from build123d import *

# Parameters (mm, degrees)
ESQUISSE1_R                  = 2.4999999999999893
ESQUISSE1_R_2                = 1.1499999999999992
EXTRUSION1_DEPTH             = 5
ESQUISSE1_R_3                = 2.5000000000000027
EXTRUSION1_2_DEPTH           = 5
EXTRUSION2_DEPTH             = 18
EXTRUSION3_DEPTH             = 2.5
ENL_V_MAT_EXTRU_1_DEPTH      = 39.32538157223775
ENL_V_MAT_EXTRU_1_DEPTH_BACK = 39.32538157223775
ESQUISSE4_R                  = 2.749999999999997
ESQUISSE4_R_2                = 2.749999999999998
CONG_3_R                     = 2
ENL_V_MAT_EXTRU_3_DEPTH      = 102.20266619760267
ENL_V_MAT_EXTRU_5_DEPTH      = 106.71602432156358
ENL_V_MAT_EXTRU_6_REACH      = 81.21
CONG_4_R                     = 6
CONG_5_R                     = 6
ESQUISSE9_R                  = 1.100000000000001
ESQUISSE9_R_2                = 1.0999999999999992
ENL_V_MAT_EXTRU_7_DEPTH      = 6


with BuildPart() as part:
    # Esquisse1 → Extrusion1 (new body)
    with BuildSketch(Plane.XY):
        with Locations((20.851873368125936, -74.73281291154764)):
            Circle(ESQUISSE1_R)
        with Locations((20.851873368125936, -74.73281291154764)):
            Circle(ESQUISSE1_R_2, mode=Mode.SUBTRACT)
    extrude(amount=EXTRUSION1_DEPTH)



with BuildPart() as body_2:
    # Esquisse1 → Extrusion1 2 (new body)
    with BuildSketch(Plane.XY):
        with Locations((-21.148126631874074, -74.73281291154764)):
            Circle(ESQUISSE1_R_3)
        with Locations((-21.148126631874074, -74.73281291154764)):
            Circle(ESQUISSE1_R_2, mode=Mode.SUBTRACT)
    extrude(amount=EXTRUSION1_2_DEPTH)


with BuildPart() as body_3:
    # Esquisse2 → Extrusion2 (new, symmetric)
    with BuildSketch(Plane(origin=(0, 0, 0), x_dir=(0, 0, -1), z_dir=(1, 0, 0))):
        Polygon((-16.664409805958893, -94.72524914650984), (-16.664409805958893, -78.97076866014885), (-7.5846798827186035, -78.97076866014885), (0, -72.23281291154765), (17.904062513857752, -57.96690094689117), (21.643440589343484, -57.97016684873832), (21.641519151826778, -60.17016600966495), (13.695222620932038, -67.54623887711948), align=None)
    extrude(amount=EXTRUSION2_DEPTH, both=True)


with BuildPart() as part_1:
    add(part.part)

    add(body_2.part)  # Extrusion3 merges body 2

    add(body_3.part)  # Extrusion3 merges body 3
    # Esquisse3 → Extrusion3 (add)
    with BuildSketch(Plane.XY.offset(2.5)):
        with BuildLine():
            Line((-23.15262617413516, -73.23883112281155), (-22.298126631874073, -73.23883112281155))
            Line((-22.298126631874073, -73.23883112281155), (-22.298126631874073, -74.73281291154764))
            ThreePointArc((-22.298126631874073, -74.73281291154764), (-21.148126631874074, -75.88281291154763), (-19.998126631874076, -74.73281291154764))
            Line((-19.998126631874076, -74.73281291154764), (-19.998126631874076, -73.23883112281155))
            Line((-19.998126631874076, -73.23883112281155), (-19.143627089612984, -73.23883112281155))
            Line((-19.143627089612984, -73.23883112281155), (-16.812156322257874, -73.23883112281158))
            Line((-16.812156322257874, -73.23883112281158), (-16.8121563222579, -77.23281291154763))
            Line((-16.8121563222579, -77.23281291154763), (-21.148126631874074, -77.23281291154764))
            ThreePointArc((-21.148126631874074, -77.23281291154764), (-23.382511834993743, -75.85420613610354), (-23.15262617413516, -73.23883112281155))
        make_face()
        with BuildLine():
            Line((18.847373825864864, -73.23883112281155), (19.701873368125938, -73.23883112281155))
            Line((19.701873368125938, -73.23883112281155), (19.701873368125938, -74.73281291154764))
            ThreePointArc((19.701873368125938, -74.73281291154764), (20.851873368125936, -75.88281291154763), (22.001873368125935, -74.73281291154764))
            Line((22.001873368125935, -74.73281291154764), (22.001873368125935, -73.23883112281155))
            Line((22.001873368125935, -73.23883112281155), (22.85637291038701, -73.23883112281155))
            ThreePointArc((22.85637291038701, -73.23883112281155), (23.0862585712456, -75.85420613610351), (20.85187336812597, -77.23281291154763))
            Line((20.85187336812597, -77.23281291154763), (16.59665054376802, -77.23281291154761))
            Line((16.59665054376802, -77.23281291154761), (16.59665054376802, -73.23883112281155))
            Line((16.59665054376802, -73.23883112281155), (18.847373825864864, -73.23883112281155))
        make_face()
    extrude(amount=EXTRUSION3_DEPTH)

    # Esquisse4 → Enlèv. mat.-Extru.1 (cut, two sides: drawn at the far end of the back side and taken through both)
    with BuildSketch(Plane(origin=(0, -78.97076866014885, 0), x_dir=(-1, 0, 0), z_dir=(0, 1, 0)).offset(-ENL_V_MAT_EXTRU_1_DEPTH_BACK)):
        with Locations(Location((-9.992794939980836, 11.38535169586409, 0), (0, 0, 270))):
            Circle(ESQUISSE4_R)
        with Locations(Location((0.00720473933372518, 11.382819165765587, 0), (0, 0, 270))):
            Circle(ESQUISSE4_R_2)
        with Locations(Location((10.007204418648286, 11.380286635667082, 0), (0, 0, 270))):
            Circle(ESQUISSE4_R_2)
    extrude(amount=ENL_V_MAT_EXTRU_1_DEPTH + ENL_V_MAT_EXTRU_1_DEPTH_BACK, mode=Mode.SUBTRACT)

    # Congé3
    cong_3_edges = [part_1.edges().sort_by_distance(p)[0] for p in [
        (-16.812156322257874, -73.23883112281158, 3.75),
        (16.59665054376802, -73.23883112281155, 3.75),
    ]]
    fillet(cong_3_edges, radius=CONG_3_R)

    # Esquisse6 → Enlèv. mat.-Extru.3 (cut, through all)
    with BuildSketch(Plane.XY.offset(5)):
        with BuildLine():
            Line((19.701873368125938, -73.23883112281155), (18.847373825864864, -73.23883112281155))
            ThreePointArc((18.847373825864864, -73.23883112281155), (20.851873368125936, -72.23281291154765), (22.85637291038701, -73.23883112281155))
            Line((22.85637291038701, -73.23883112281155), (22.001873368125935, -73.23883112281155))
            Line((22.001873368125935, -73.23883112281155), (22.001873368125935, -74.73281291154764))
            ThreePointArc((22.001873368125935, -74.73281291154764), (20.851873368125936, -75.88281291154763), (19.701873368125938, -74.73281291154764))
            Line((19.701873368125938, -74.73281291154764), (19.701873368125938, -73.23883112281155))
        make_face()
        with BuildLine():
            Line((-19.143627089612988, -73.23883112281155), (-19.998126631874076, -73.23883112281155))
            Line((-19.998126631874076, -73.23883112281155), (-19.998126631874076, -74.73281291154764))
            ThreePointArc((-19.998126631874076, -74.73281291154764), (-21.148126631874074, -75.88281291154763), (-22.298126631874073, -74.73281291154764))
            Line((-22.298126631874073, -74.73281291154764), (-22.298126631874073, -73.23883112281155))
            Line((-22.298126631874073, -73.23883112281155), (-23.15262617413516, -73.23883112281155))
            ThreePointArc((-23.15262617413516, -73.23883112281155), (-21.148126631874074, -72.23281291154764), (-19.143627089612988, -73.23883112281155))
        make_face()
    extrude(amount=-ENL_V_MAT_EXTRU_3_DEPTH, mode=Mode.SUBTRACT)

    # Esquisse7 → Enlèv. mat.-Extru.5 (cut, through all)
    with BuildSketch(Plane(origin=(18, 0, 0), x_dir=(0, 0, -1), z_dir=(1, 0, 0))):
        Polygon((22.38759689084557, -59.06637403320253), (18.619915990338253, -59.06637403320253), (2.127272735037141, -72.00940646483387), (2.127272735037142, -79.68956966642843), (22.38759689084557, -60.215467045024496), align=None)
    extrude(amount=-ENL_V_MAT_EXTRU_5_DEPTH, mode=Mode.SUBTRACT)

    # Enlèv. mat.-Extru.6: up to this plane
    enl_v_mat_extru_6_end = Plane(origin=(-23.648126631874074, -59.06637403320253, -18.619915990338253), z_dir=(0, 0.7866767496715903, 0.6173651201081433))
    # Esquisse8 → Enlèv. mat.-Extru.6 (cut, up to the surface)
    with BuildSketch(Plane(origin=(0, -44.301458010279546, -39.66022266935793), x_dir=(1, 0, 0), z_dir=(0, -0.745056791328178, -0.6670010327546427)), mode=Mode.PRIVATE) as enl_v_mat_extru_6_sk1:
        Polygon((16.22439568808015, 59.743411480582274), (-16.434037279491676, 59.74341148058227), (-16.43403727949168, 40.55997816141156), (16.22439568808015, 40.559978161411564), align=None)
    enl_v_mat_extru_6_tool1 = split(extrude(enl_v_mat_extru_6_sk1.sketch, amount=-ENL_V_MAT_EXTRU_6_REACH, mode=Mode.PRIVATE), bisect_by=enl_v_mat_extru_6_end, keep=Keep.BOTH, mode=Mode.PRIVATE)
    add(enl_v_mat_extru_6_tool1.solids().sort_by_distance((-0.104821, -77.75269, -2.294362))[0], mode=Mode.SUBTRACT)

    # Congé4
    cong_4_edges = [part_1.edges().sort_by_distance(p)[0] for p in [
        (-17.217018639745838, -77.90227429690431, -2.127272735037141),
        (17.112197844040075, -77.90227429690431, -2.127272735037141),
    ]]
    fillet(cong_4_edges, radius=CONG_4_R)

    # Congé5
    cong_5_edges = [part_1.edges().sort_by_distance(p)[0] for p in [
        (-18, -86.84800890332934, 16.664409805958893),
        (18, -86.84800890332934, 16.664409805958893),
    ]]
    fillet(cong_5_edges, radius=CONG_5_R)

    # Esquisse9 → Enlèv. mat.-Extru.7 (cut)
    with BuildSketch(Plane(origin=(0, -78.97076866014885, 0), x_dir=(-1, 0, 0), z_dir=(0, 1, 0))):
        with Locations(Location((-16, 9.584679882718603, 0), (0, 0, 90))):
            Circle(ESQUISSE9_R)
        with Locations(Location((16, 9.584679882718603, 0), (0, 0, 90))):
            Circle(ESQUISSE9_R_2)
    extrude(amount=-ENL_V_MAT_EXTRU_7_DEPTH, mode=Mode.SUBTRACT)


solid = part_1.part
Build history of the part. All positions in model axes, mm. A direction names the side the tool comes from. Give positions to 0.01 mm unless a question says otherwise; leave off trailing zeros. Order: outer loops, then holes, each group sorted by start corner. A loop starts at its lowest first (then second) coordinate and runs counter-clockwise, first axis right, second up. Notation, with made-up numbers: M 20,39.5 L 35,39.5 A31 cw 35,78.5 Z; hole C 2,84 d6. An arc over 180 degrees is marked long. Use one line per item in the form item = value.
Q1. Wall check: probe 1 along X at (y, z) = (-80, 11); probe 2 along Y at (x, z) = (5.5, 5.5); probe 3 along Z at (x, y) = (-10, -80). Give the ranges that are in metal, low to high.
Conclusion:
probe_1 = -17.99 to -12.73, -7.28 to -2.73, 2.72 to 7.27, 12.72 to 17.99
probe_2 = -84.73 to -83.43, -78 to -77.12
probe_3 = 8.05 to 8.63, 14.13 to 16.66
Q2. Pin check, flat tips, straight feed: P1, Ø10, axis at x = -0.5, y = -71.5, coming from the +Z side; P2, Ø8, axis at x = -6.5, z = 6.5, coming from the -Y side; P3, Ø2.5, axis at x = -16, z = 9.58, coming from the +Y side; P4, Ø12, axis at y = -73.5, z = -4.5, coming from the -X side. Stop position of each tip, or through.
Conclusion:
P1 = 4.8
P2 = -89.21
P3 = -78.97
P4 = -23.65
Q3. Pull direction Z, two halves, no side cores. Call faces 1 (the flat face through (-17, -74, -2.127)), 2 (the flat face through (0, -87, 16.664)), 3 (the cylindrical face through (-0.13, -84.35, 14.13)): released by +Z, released by -Z, zero draft, split by the parting line, or undercut.
Conclusion:
face_1 = released by -Z
face_2 = released by +Z
face_3 = undercut
Q4. Slice it at A-A, the plane x = -8. Write the cut outline in (y, z).
Conclusion:
outline = M -94.73,16.66 L -91.68,13.26 L -78.97,13.26 L -78.97,16.66 Z; M -88.31,9.5 L -84.15,4.85 L -80.24,8.36 L -59.07,-18.62 L -59.07,-21.64 L -57.97,-21.64 L -57.97,-17.9 L -72.23,0 L -78.97,7.58 L -78.97,9.5 Z
Q5. Which spindle directions (+Z, -Z, +X, -X, +Y, -Y) get a long thin tool onto all of the face, cutting with end or side? Do faces 4 (the flat face through (0, -59.066, -20)), 5 (the flat face through (19, -77.233, 4)), 6 (the flat face through (0, -78.971, 15)), 7 (the flat face through (20.8, -76.1, 0)), 8 (the flat face through (-16.434, -79, 3)). Say none if no direction does.
Conclusion:
face_4 = -Z, +X, -X, -Y
face_5 = +Z, -Z, +X, -Y
face_6 = +Z, +X, -X, +Y
face_7 = -Z, +X, +Y, -Y
face_8 = -Z
Q6. Slice it at B-B, the plane z = 12. Write the cut outline in (x, y).
Conclusion:
outline = M -17.85,-90.55 L -12.69,-90.55 L -12.69,-78.97 L -17.85,-78.97 Z; M -7.33,-90.55 L -2.69,-90.55 L -2.69,-78.97 L -7.33,-78.97 Z; M 2.67,-90.55 L 7.31,-90.55 L 7.31,-78.97 L 2.67,-78.97 Z; M 12.67,-90.55 L 17.85,-90.55 L 17.85,-78.97 L 12.67,-78.97 Z
Q7. Slice it at D-D, the plane x = 8. Write the cut outline in (y, z), and give its area (3 significant figures).
Conclusion:
outline = M -94.73,16.66 L -91.7,13.28 L -78.97,13.28 L -78.97,16.66 Z; M -88.3,9.49 L -84.15,4.85 L -80.24,8.36 L -59.07,-18.62 L -59.07,-21.64 L -57.97,-21.64 L -57.97,-17.9 L -72.23,0 L -78.97,7.58 L -78.97,9.49 Z
area = 111 mm2
Q8. Slice it at C-C, the plane y = -83. Write the cut outline in (x, z), and give its area (3 significant figures).
Conclusion:
outline = M -18,3.57 L -16.43,3.57 L -16.43,5.88 L 16.22,5.88 L 16.22,3.57 L 18,3.57 L 18,10.66 A6 ccw 12,16.66 L -12,16.66 A6 ccw -18,10.66 Z; hole C -16,9.58 d2.2; hole C -10.01,11.38 d5.5; hole C -0.01,11.38 d5.5; hole C 9.99,11.39 d5.5; hole C 16,9.58 d2.2
area = 302 mm2
